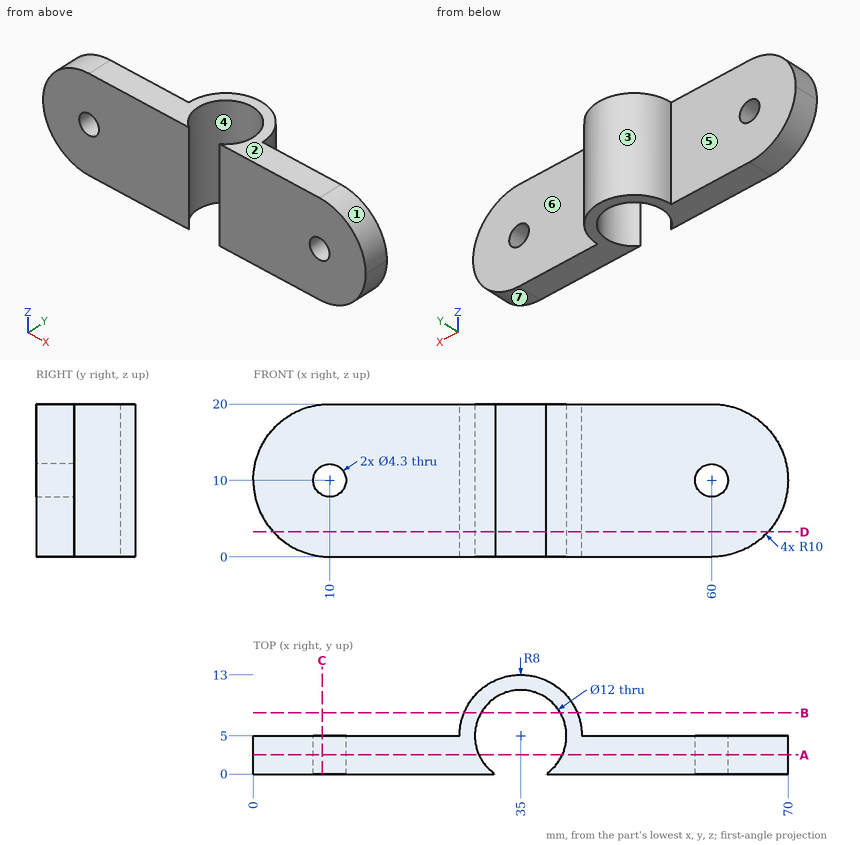
Input: dimensioned drawing with shaded views. Units: mm. Origin: part minimum x, y, z. A direction names the side the tool comes from. Coordinates: 2 decimals unless noted, no trailing zeros. Write each loop counter-clockwise with the first axis right and the second up, starting at its lowest first coordinate (ties: lowest second). Pieces come first, ordered by that corner, then holes. Notation, with made-up numbers: M 6.25,59.25 L 55.25,59.25 A15 ccw 55.25,86.25 Z; hole C -14,19 d2. An arc over 180 degrees is marked long. Use one line per item in the form item = value.
Q1. Section B-B (y = 8). Return loops of the section in (x, z).
Answer below:
outline = M 27.58,0 L 29.8,0 L 29.8,20 L 27.58,20 Z; M 40.2,0 L 42.42,0 L 42.42,20 L 40.2,20 Z
Q2. Section A-A (y = 2.5). Count the separate pieces of the cut face and the enclosed holes in it, plus the area to 3 significant figures.
Answer below:
separate_pieces = 2
enclosed_holes = 2
area = 1,070 mm²
Q3. Material intervals for probe 1 along X at (y, z) = (3.5, 10); probe 2 along X at (y, z) = (1.6, 10); probe 3 along Z at (x, y) = (60, 2.3), sorted ascending. Write a range as from..to.
Answer below:
probe_1 = 0..7.85, 12.15..29.19, 40.81..57.85, 62.15..70
probe_2 = 0..7.85, 12.15..30.06, 39.94..57.85, 62.15..70
probe_3 = 0..7.85, 12.15..20
Q4. Section D-D (z = 3.25). Return loops of the section in (x, y).
Answer below:
outline = M 2.62,0 L 31.68,0 A6 cw long 38.32,0 L 67.38,0 L 67.38,5 L 43,5 A8 ccw 27,5 L 2.62,5 Z
Q5. First-contact query: pin 1 (6 mm diameter, centred on x = 54, z = 10, fed in from +Y). Flat tip, straight axial feed; report the tip coordinate or a pass-through.
Answer below:
pin_1 = 5
Q6. Set-up query: the marked faces 5, 6 and 7. Return all of +Z, -Z, +X, -X, +Y, -Y with unobstructed straight access to the full face (end or side cutting, diameter ignored); none if empty.
Answer below:
face_5 = +Z, -Z, -X, +Y
face_6 = +Z, -Z, +X, +Y
face_7 = -Z, +X, +Y, -Y
Q7. Draft query along X for the marked faces 1, 2, 3 and 4. Return one class per face: released by +X, released by -X, zero draft, split by the parting line, or undercut.
Answer below:
face_1 = released by +X
face_2 = zero draft
face_3 = split by the parting line
face_4 = undercut
Q8. Section C-C (x = 9). Return loops of the section in (y, z).
Answer below:
outline = M 0,0.05 L 5,0.05 L 5,8.1 L 0,8.1 Z; M 0,11.9 L 5,11.9 L 5,19.95 L 0,19.95 Z
